Could you check a few things on this model? Use its own coordinates, in mm. A direction names the side the tool comes from. Give positions to 0.01 mm unless a question says otherwise; leave off trailing zeros. Loops run counter-clockwise (first coordinate to the right, second up) from the corner with the lowest first, then second, coordinate; pieces in that order, holes last. Notation, with made-up numbers: (-22.5, -4) - (13.5, -4) arc R15 cw to (13.5, 3) - close; hole circle Ø9 at (49, -31.5). An arc over 180 degrees is marked (long way). Write each question's results on one line, items separated by ' | '. Start each with the question number.
(1) Suppose I cut it at B-B (z = 5.5). Please give me the cut outline in (x, y), and give its area (3 significant figures).
(2) I need wall thicknesses on line 1 (Y direction, x = 18.5, z = -1); line 2 (Y direction, x = 30, z = 3.25); line 3 (Z direction, x = -16.5, y = -10). Which ranges of each line are inside material? Lowest first, please.
(3) On a 3-axis mill with a long thin cutter (end or side, diameter ignored), from which of +Z, -Z, +X, -X, +Y, -Y can I reach the whole of each face in a straight line? I mean faces 1 (the face through (-35.4, -19.43, 10.11)), 2 (the face through (1, -25.1, -1)), 3 (the face through (-1, -25.1, 6)), 4 (the face through (40, 0, 6)). Say none if no direction works.
(4) For pin 1 (1.2 mm diameter, centred on y = 23.5, z = -2, fed in from -X); pin 2 (0.8 mm diameter, centred on x = 2.5, z = 10, fed in from -Y); pin 3 (3.5 mm diameter, centred on x = 14.5, z = -1, fed in from -Y); pin 4 (2.5 mm diameter, centred on x = 19, z = -2, fed in from +Y), each with a flat end and sliding along its axis, tell me the tip position at first contact or that it passes through.
(5) Suppose I cut it at A-A (x = 2). Please give me the cut outline in (y, z).
(6) Suppose I cut it at C-C (x = 46.5). Please give me the cut outline in (y, z), and give its area (3 significant figures).
(7) If we mould it in two halves opening along X, with no side actions, what happens to faces 5 (the face through (-40, 0, 6)), 6 (the face through (-1, 25.1, 6)), 7 (the face through (55.6, -21.8, 0.8))? For each: released by +X, released by -X, zero draft, split by the parting line, or undercut.
from build123d import *

# Parameters (mm, degrees)
ESQUISSE1_W             = 113
ESQUISSE1_H             = 53
ESQUISSE1_R             = 2
ESQUISSE1_R_2           = 0.5
BOSS_EXTRU_1_DEPTH      = 1.6
ESQUISSE2_W             = 80
ESQUISSE2_H             = 50.2
BOSS_EXTRU_2_DEPTH      = 9
ENL_V_MAT_EXTRU_1_DEPTH = 1
ESQUISSE6_W             = 80
ESQUISSE6_H             = 2.428445289
ESQUISSE6_H_2           = 1.774946784
BOSS_EXTRU_3_DEPTH      = 3


with BuildPart() as part:
    # Esquisse1 → Boss.-Extru.1 (new body)
    with BuildSketch(Plane.XY):
        Rectangle(ESQUISSE1_W, ESQUISSE1_H)
        with Locations((-54, 23)):
            Circle(ESQUISSE1_R, mode=Mode.SUBTRACT)
        with Locations((-54, -23)):
            Circle(ESQUISSE1_R, mode=Mode.SUBTRACT)
        with Locations(Location((54, -23, 0), (0, 0, 180))):
            Circle(ESQUISSE1_R, mode=Mode.SUBTRACT)
        with Locations(Location((54, 23, 0), (0, 0, 180))):
            Circle(ESQUISSE1_R, mode=Mode.SUBTRACT)
        with Locations((-54, 11.43)):
            Circle(ESQUISSE1_R_2, mode=Mode.SUBTRACT)
        with Locations((-51.46, 11.43)):
            Circle(ESQUISSE1_R_2, mode=Mode.SUBTRACT)
        with Locations((-51.46, 8.89)):
            Circle(ESQUISSE1_R_2, mode=Mode.SUBTRACT)
        with Locations((-51.46, 6.35)):
            Circle(ESQUISSE1_R_2, mode=Mode.SUBTRACT)
        with Locations((-51.46, 3.81)):
            Circle(ESQUISSE1_R_2, mode=Mode.SUBTRACT)
        with Locations((-51.46, 1.27)):
            Circle(ESQUISSE1_R_2, mode=Mode.SUBTRACT)
        with Locations((-51.46, -1.27)):
            Circle(ESQUISSE1_R_2, mode=Mode.SUBTRACT)
        with Locations((-51.46, -3.81)):
            Circle(ESQUISSE1_R_2, mode=Mode.SUBTRACT)
        with Locations((-51.46, -6.35)):
            Circle(ESQUISSE1_R_2, mode=Mode.SUBTRACT)
        with Locations((-51.46, -8.89)):
            Circle(ESQUISSE1_R_2, mode=Mode.SUBTRACT)
        with Locations((-51.46, -11.43)):
            Circle(ESQUISSE1_R_2, mode=Mode.SUBTRACT)
        with Locations((-54, 8.89)):
            Circle(ESQUISSE1_R_2, mode=Mode.SUBTRACT)
        with Locations((-54, 6.35)):
            Circle(ESQUISSE1_R_2, mode=Mode.SUBTRACT)
        with Locations((-54, 3.81)):
            Circle(ESQUISSE1_R_2, mode=Mode.SUBTRACT)
        with Locations((-54, 1.27)):
            Circle(ESQUISSE1_R_2, mode=Mode.SUBTRACT)
        with Locations((-54, -1.27)):
            Circle(ESQUISSE1_R_2, mode=Mode.SUBTRACT)
        with Locations((-54, -3.81)):
            Circle(ESQUISSE1_R_2, mode=Mode.SUBTRACT)
        with Locations((-54, -6.35)):
            Circle(ESQUISSE1_R_2, mode=Mode.SUBTRACT)
        with Locations((-54, -8.89)):
            Circle(ESQUISSE1_R_2, mode=Mode.SUBTRACT)
        with Locations((-54, -11.43)):
            Circle(ESQUISSE1_R_2, mode=Mode.SUBTRACT)
    extrude(amount=BOSS_EXTRU_1_DEPTH)

    # Esquisse2 → Boss.-Extru.2 (add)
    with BuildSketch(Plane.XY.offset(1.6)):
        Rectangle(ESQUISSE2_W, ESQUISSE2_H)
    extrude(amount=BOSS_EXTRU_2_DEPTH)

    # Esquisse4 → Enlèv. mat.-Extru.1 (cut)
    with BuildSketch(Plane.XY.offset(10.6)):
        with BuildLine():
            Line((34, -20), (-34, -20))
            ThreePointArc((-34, -20), (-35.414213562, -19.414213562), (-36, -18))
            Line((-36, -18), (-36, 18))
            ThreePointArc((-36, 18), (-35.414213562, 19.414213562), (-34, 20))
            Line((-34, 20), (34, 20))
            ThreePointArc((34, 20), (35.414213562, 19.414213562), (36, 18))
            Line((36, 18), (36, -18))
            ThreePointArc((36, -18), (35.414213562, -19.414213562), (34, -20))
        make_face()
    extrude(amount=-ENL_V_MAT_EXTRU_1_DEPTH, mode=Mode.SUBTRACT)

    # Esquisse6 → Boss.-Extru.3 (add)
    with BuildSketch(Plane(origin=(0, 0, 0), x_dir=(-1, 0, 0), z_dir=(0, 0, -1))):
        with Locations((0, 23.885777356)):
            Rectangle(ESQUISSE6_W, ESQUISSE6_H)
        with Locations((0, -24.212526608)):
            Rectangle(ESQUISSE6_W, ESQUISSE6_H_2)
    extrude(amount=BOSS_EXTRU_3_DEPTH)


solid = part.part
Output values:
1) outline: (-40, -25.1) - (40, -25.1) - (40, 25.1) - (-40, 25.1) - close | area: 4,020 mm2
2) line 1: -25.1 to -23.33, 22.67 to 25.1 | line 2: -25.1 to 25.1 | line 3: 0 to 9.6
3) face 1: +Z | face 2: -Z, +X, -X, -Y | face 3: +Z, +X, -X, -Y | face 4: +Z, +X, +Y, -Y
4) pin 1: x = -40 | pin 2: y = -25.1 | pin 3: y = -26.5 | pin 4: y = 25.1
5) outline: (-26.5, 0) - (-25.1, 0) - (-25.1, -3) - (-23.33, -3) - (-23.33, 0) - (22.67, 0) - (22.67, -3) - (25.1, -3) - (25.1, 0) - (26.5, 0) - (26.5, 1.6) - (25.1, 1.6) - (25.1, 10.6) - (20, 10.6) - (20, 9.6) - (-20, 9.6) - (-20, 10.6) - (-25.1, 10.6) - (-25.1, 1.6) - (-26.5, 1.6) - close
6) outline: (-26.5, 0) - (26.5, 0) - (26.5, 1.6) - (-26.5, 1.6) - close | area: 84.8 mm2
7) face 5: released by -X | face 6: zero draft | face 7: undercut
